For this review, take the finished solid that the model builds, in its own axes (mm). Face numbers are marked on the shaded views. A direction names the side the tool comes from. Coordinates: 2 decimals unless noted, no trailing zeros. Order: outer loops, then holes, each group sorted by start corner. A loop starts at its lowest first (then second) coordinate and runs counter-clockwise, first axis right, second up. Notation, with made-up numbers: (-14, 55.5) -> (41, 55.5) arc R24 cw to (41, 94.5) -> close; hole circle Ø3 at (-30, -29). An arc over 180 degrees is marked (long way). Return JSON: item names as keys, results as strings. Group by question number.
Item 1: Machinability: for the marked faces 1 and 2, which of the approach directions +Z, -Z, +X, -X, +Y, -Y give a long, thin tool a straight path to every point of the face, cutting with its end or side? Answer none if there is none.
Item 2: Take a section at C-C (y = 5). Write out the cut boundary in (x, z) (1 decimal).
Item 3: Take a section at D-D (y = 1.75). Count the separate pieces of the cut face and the enclosed holes in it, then the cut area to 3 significant figures.
Item 4: For line 1 along X through (y, z) = (2.7, 0); line 2 along Z through (x, y) = (0, 5.5) (1 decimal); line 3 along X through (y, z) = (7.5, 0), list the stretches that pass through material, from the lowest coordinate up.
Item 5: Insertion check: pin 1 (3 mm diameter, centred on x = -7, y = 2.5, fed in from -Z); pin 2 (6 mm diameter, centred on y = 7, z = -15.5, fed in from +X); pin 3 (2.5 mm diameter, centred on x = 0, z = -18.415, fed in from +Y); pin 4 (5 mm diameter, centred on x = 0, z = 20.64, fed in from +Y). Each pin has a flat end and moves straight along its axis. Give the tip position at first contact, or say it passes through.
Item 6: Take a section at B-B (z = 0). Write out the cut boundary in (x, y), then the cut area to 3 significant figures.
Item 7: Draft analysis for pull direction Z (two halves, no side actions). For the marked faces 3, 4 and 5, state which applies: +Z half, -Z half, draft (parallel to the pull), parting line (faces both ways), or undercut.
Item 8: Take a section at A-A (x = 0). Write out the cut boundary in (y, z) (1 decimal).
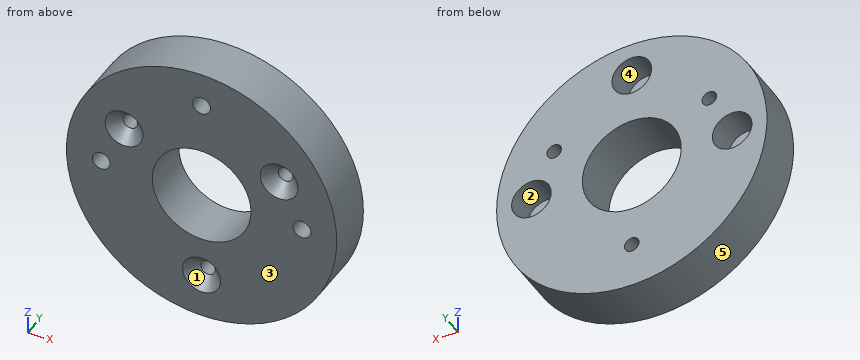
```python
from build123d import *

# Parameters (mm, degrees)
SKETCH1_R               = 27.7876
SKETCH1_R_2             = 10.16
RING_DEPTH              = 10
SKETCH2_R               = 1.5
ROBOT_SIDE1_HOLES_DEPTH = 11
ROBOT_SIDE_CHAMFER_SIZE = 2.4
SKETCH3_R               = 1.838724863
TOOL_SIDE_HOLES_DEPTH   = 11
SKETCH4_R               = 4.064
TOOL_SIDE_INSET_DEPTH   = 6


with BuildPart() as part:
    # Sketch1 → Ring (new body)
    with BuildSketch(Plane(origin=(0, 0, 0), x_dir=(1, 0, 0), z_dir=(0, 1, 0))):
        Circle(SKETCH1_R)
        Circle(SKETCH1_R_2, mode=Mode.SUBTRACT)
    extrude(amount=RING_DEPTH)

    # Sketch2 → Robot Side1 - Holes (cut, through all)
    with BuildSketch(Plane(origin=(0, 10, 0), x_dir=(1, 0, 0), z_dir=(0, 1, 0))):
        with Locations((0, 18.415)):
            Circle(SKETCH2_R)
        with Locations((15.947857811, -9.2075)):
            Circle(SKETCH2_R)
        with Locations((-15.947857811, -9.2075)):
            Circle(SKETCH2_R)
    extrude(amount=-ROBOT_SIDE1_HOLES_DEPTH, mode=Mode.SUBTRACT)

    # Robot Side - Chamfer
    robot_side_chamfer_edges = [part.edges().sort_by_distance(p)[0] for p in [
        (-1.5, 0, -18.415),
        (14.447857811, 0, 9.2075),
        (-17.447857811, 0, 9.2075),
    ]]
    chamfer(robot_side_chamfer_edges, length=ROBOT_SIDE_CHAMFER_SIZE)

    # Sketch3 → Tool Side - Holes (cut, through all)
    with BuildSketch(Plane(origin=(0, 10, 0), x_dir=(1, 0, 0), z_dir=(0, 1, 0))):
        with Locations((20.6375, 0)):
            Circle(SKETCH3_R)
        with Locations((0, -20.6375)):
            Circle(SKETCH3_R)
        with Locations((-20.6375, 0)):
            Circle(SKETCH3_R)
    extrude(amount=-TOOL_SIDE_HOLES_DEPTH, mode=Mode.SUBTRACT)

    # Sketch4 → Tool Side - Inset (cut)
    with BuildSketch(Plane(origin=(0, 10, 0), x_dir=(1, 0, 0), z_dir=(0, 1, 0))):
        with Locations((-20.6375, 0)):
            Circle(SKETCH4_R)
        with Locations((0, -20.6375)):
            Circle(SKETCH4_R)
        with Locations((20.6375, 0)):
            Circle(SKETCH4_R)
    extrude(amount=-TOOL_SIDE_INSET_DEPTH, mode=Mode.SUBTRACT)


solid = part.part
```
Findings below:
{
 "1": {"face 1": "-Y", "face 2": "+Y"},
 "2": {"outline": "circle Ø55.6 at (0, 0); hole circle Ø8.1 at (-20.6, 0); hole circle Ø3 at (-15.9, 9.2); hole circle Ø20.3 at (0, 0); hole circle Ø8.1 at (0, 20.6); hole circle Ø3 at (0, -18.4); hole circle Ø3 at (15.9, 9.2); hole circle Ø8.1 at (20.6, 0)"},
 "3": {"separate pieces": "1", "enclosed holes": "7", "area": "2,030 mm2"},
 "4": {"line 1": "x = -27.79 to -22.48, -18.8 to -10.16, 10.16 to 18.8, 22.48 to 27.79", "line 2": "z = -27.8 to -19.9, -16.9 to -10.2, 10.2 to 16.6, 24.7 to 27.8", "line 3": "x = -27.79 to -24.7, -16.57 to -10.16, 10.16 to 16.57, 24.7 to 27.79"},
 "5": {"pin 1": "stops at z = -27.24", "pin 2": "stops at x = 24.82", "pin 3": "passes through", "pin 4": "stops at y = 4"},
 "6": {"outline": "(-27.79, 0) -> (-22.48, 0) -> (-22.48, 4) -> (-24.7, 4) -> (-24.7, 10) -> (-27.79, 10) -> close; (-18.8, 0) -> (-10.16, 0) -> (-10.16, 10) -> (-16.57, 10) -> (-16.57, 4) -> (-18.8, 4) -> close; (10.16, 0) -> (18.8, 0) -> (18.8, 4) -> (16.57, 4) -> (16.57, 10) -> (10.16, 10) -> close; (22.48, 0) -> (27.79, 0) -> (27.79, 10) -> (24.7, 10) -> (24.7, 4) -> (22.48, 4) -> close", "area": "226 mm2"},
 "7": {"face 3": "draft", "face 4": "undercut", "face 5": "parting line"},
 "8": {"outline": "(0, -27.8) -> (10, -27.8) -> (10, -19.9) -> (2.4, -19.9) -> (0, -22.3) -> close; (0, -14.5) -> (2.4, -16.9) -> (10, -16.9) -> (10, -10.2) -> (0, -10.2) -> close; (0, 10.2) -> (10, 10.2) -> (10, 16.6) -> (4, 16.6) -> (4, 18.8) -> (0, 18.8) -> close; (0, 22.5) -> (4, 22.5) -> (4, 24.7) -> (10, 24.7) -> (10, 27.8) -> (0, 27.8) -> close"}
}
